Autodesk Inventor part; units mm, degrees
ref_plane "Work Plane1" through (0, 0, 5) normal (0, 0, 1) x (1, 0, 0)
ref_plane "YZ Plane" through (0, 0, 0) normal (1, 0, 0) x (0, 1, 0)
ref_plane "XZ Plane" through (0, 0, 0) normal (0, 1, 0) x (-1, 0, 0)
sketch "Sketch1" plane through (0, 0, 0) normal (0, 0, 1) x (1, 0, 0)
  line L0 (14.6962, 12.74) -> (14.6962, 0) construction
  line L1 (10.61, 12.2) -> (1.53, 12.2)
  arc A0 (1.53, 12.2) -> (0, 10.67) centre (1.53, 10.67) ccw
  line L2 (0, 10.67) -> (0, 1.53)
  arc A1 (0, 1.53) -> (1.53, 0) centre (1.53, 1.53) ccw
  line L3 (1.53, 0) -> (10.61, 0)
  arc A2 (10.61, 0) -> (12.14, 1.53) centre (10.61, 1.53) ccw
  arc A3 (12.14, 10.67) -> (10.61, 12.2) centre (10.61, 10.67) ccw
  line L4 (12.14, 10.67) -> (12.14, 1.53)
  point P0 (0, 0)
  point P1 (0, 0)
  dimension "d10" = 12.74
ref_plane "Work Plane1" through (0, 0, 5) normal (0, 0, 1) x (1, 0, 0)
sketch "Sketch2" plane through (0, 0, 5) normal (0, 0, 1) x (1, 0, 0)
  line L0 (10.88, 12.74) -> (1.8, 12.74)
  line L1 (10.88, 12.74) -> (1.8, 12.74)
  arc A0 (1.8, 12.74) -> (0, 10.94) centre (1.8, 10.94) ccw
  line L2 (0, 10.94) -> (0, 1.8)
  arc A1 (0, 1.8) -> (1.8, 0) centre (1.8, 1.8) ccw
  line L3 (1.8, 0) -> (10.88, 0)
  arc A2 (10.88, 0) -> (12.68, 1.8) centre (10.88, 1.8) ccw
  line L4 (12.68, 1.8) -> (12.68, 10.94)
  arc A3 (12.68, 10.94) -> (10.88, 12.74) centre (10.88, 10.94) ccw
  circle A4 centre (6.34, 6.37) radius 2.8
  line L5 (5.665, 8.395) -> (7.015, 8.395)
  line L6 (7.015, 4.345) -> (5.665, 4.345)
  line L7 (5.665, 4.345) -> (7.015, 8.395) construction
  line L8 (5.665, 8.395) -> (7.015, 4.345) construction
  line L9 (8.365, 5.695) -> (8.365, 7.045)
  line L10 (4.315, 7.045) -> (4.315, 5.695)
  line L11 (4.315, 5.695) -> (8.365, 7.045) construction
  line L12 (8.365, 5.695) -> (4.315, 7.045) construction
  line L13 (4.315, 5.695) -> (5.665, 5.695)
  line L14 (7.015, 5.695) -> (8.365, 5.695)
  line L15 (5.665, 4.345) -> (5.665, 5.695)
  line L16 (5.665, 7.045) -> (5.665, 8.395)
  line L17 (8.365, 7.045) -> (7.015, 7.045)
  line L18 (5.665, 7.045) -> (4.315, 7.045)
  line L19 (7.015, 8.395) -> (7.015, 7.045)
  line L20 (7.015, 5.695) -> (7.015, 4.345)
  point P0 (0, 0)
  dimension "d12" = 5
  dimension "d3" = 5.6
  dimension "d4" = 4.05
  dimension "d5" = 1.35
  dimension "d6" = 4.05
  dimension "d7" = 1.35
extrude "Extrusion3" add sketch "Sketch1" along normal blind 5
sketch "Sketch3" plane through (0, 0, 5) normal (0, 0, 1) x (1, 0, 0)
  line L0 (10.61, 12.47) -> (1.53, 12.47)
  line L1 (10.61, 12.47) -> (1.53, 12.47)
  arc A0 (1.53, 12.47) -> (-0.27, 10.67) centre (1.53, 10.67) ccw
  line L2 (-0.27, 10.67) -> (-0.27, 1.53)
  arc A1 (-0.27, 1.53) -> (1.53, -0.27) centre (1.53, 1.53) ccw
  line L3 (1.53, -0.27) -> (10.61, -0.27)
  arc A2 (10.61, -0.27) -> (12.41, 1.53) centre (10.61, 1.53) ccw
  line L4 (12.41, 1.53) -> (12.41, 10.67)
  arc A3 (12.41, 10.67) -> (10.61, 12.47) centre (10.61, 10.67) ccw
  circle A4 centre (6.07, 6.1) radius 2.8
  line L5 (5.395, 8.125) -> (6.745, 8.125)
  line L6 (6.745, 4.075) -> (5.395, 4.075)
  line L7 (5.395, 4.075) -> (6.745, 8.125) construction
  line L8 (5.395, 8.125) -> (6.745, 4.075) construction
  line L9 (8.095, 5.425) -> (8.095, 6.775)
  line L10 (4.045, 6.775) -> (4.045, 5.425)
  line L11 (4.045, 5.425) -> (8.095, 6.775) construction
  line L12 (8.095, 5.425) -> (4.045, 6.775) construction
  line L13 (4.045, 5.425) -> (5.395, 5.425)
  line L14 (6.745, 5.425) -> (8.095, 5.425)
  line L15 (5.395, 4.075) -> (5.395, 5.425)
  line L16 (5.395, 6.775) -> (5.395, 8.125)
  line L17 (8.095, 6.775) -> (6.745, 6.775)
  line L18 (5.395, 6.775) -> (4.045, 6.775)
  line L19 (6.745, 8.125) -> (6.745, 6.775)
  line L20 (6.745, 5.425) -> (6.745, 4.075)
  line L21 (10.61, 12.2) -> (1.53, 12.2)
  line L22 (0, 10.67) -> (0, 1.53)
  point P0 (0, 0)
  point P1 (-0.27, -0.27)
  point P2 (6.07, 12.2)
  point P3 (0, 6.1)
  point P4 (6.07, 6.1)
  dimension "d14" = 5.6
  dimension "d15" = 4.05
  dimension "d16" = 1.35
  dimension "d17" = 4.05
  dimension "d18" = 1.35
extrude "Extrusion4" add sketch "Sketch3" along normal blind 4.8 contours A4
sketch "Sketch4" plane through (0, 0, 0) normal (0, 0, -1) x (-1, 0, 0)
  line L0 (-13.9436, 0) -> (-13.9436, 2.266)
  line L1 (-15.5559, 0) -> (-15.5559, 6.84)
  line L2 (-1.53, 0) -> (-10.61, 0)
  line L3 (-11.3457, 9.9988) -> (-0.7943, 9.9988) construction
  line L4 (-0.7943, 9.9988) -> (-0.7943, 6.84) construction
  line L5 (-0.7943, 6.84) -> (-11.3457, 6.84) construction
  line L6 (-11.3457, 6.84) -> (-11.3457, 9.9988) construction
  line L7 (-7.4059, 5.3234) -> (-4.7341, 5.3234) construction
  line L8 (-4.7341, 5.3234) -> (-4.7341, 2.266) construction
  line L9 (-4.7341, 2.266) -> (-7.4059, 2.266) construction
  line L10 (-7.4059, 2.266) -> (-7.4059, 5.3234) construction
  spline S0 degree 2 poles (-10.0876, 6.84) (-10.4386, 6.84) (-10.9675, 6.9759) (-11.1949, 7.0748) knots 0 0 0 1 2 2 2
  line L11 (-11.1949, 7.0748) -> (-11.1949, 7.8015)
  line L12 (-11.1949, 7.8015) -> (-11.1257, 7.8015)
  spline S1 degree 2 poles (-11.1257, 7.8015) (-10.8959, 7.6062) (-10.3447, 7.3961) (-10.0852, 7.3961) knots 0 0 0 1 2 2 2
  spline S2 degree 2 poles (-10.0852, 7.3961) (-10.0184, 7.3961) (-9.8034, 7.4258) (-9.7391, 7.4554) knots 0 0 0 1 2 2 2
  spline S3 degree 2 poles (-9.7391, 7.4554) (-9.6601, 7.49) (-9.5488, 7.6161) (-9.5488, 7.7174) knots 0 0 0 1 2 2 2
  spline S4 degree 2 poles (-9.5488, 7.7174) (-9.5488, 7.8336) (-9.7293, 7.977) (-9.8528, 8.0091) knots 0 0 0 1 2 2 2
  spline S5 degree 2 poles (-9.8528, 8.0091) (-10.0086, 8.0511) (-10.362, 8.1228) (-10.5177, 8.1772) knots 0 0 0 1 2 2 2
  spline S6 degree 2 poles (-10.5177, 8.1772) (-10.8712, 8.3007) (-11.1776, 8.7234) (-11.1776, 9.0398) knots 0 0 0 1 2 2 2
  spline S7 degree 2 poles (-11.1776, 9.0398) (-11.1776, 9.4674) (-10.4534, 9.9988) (-9.9097, 9.9988) knots 0 0 0 1 2 2 2
  spline S8 degree 2 poles (-9.9097, 9.9988) (-9.6378, 9.9988) (-9.099, 9.8875) (-8.8864, 9.7936) knots 0 0 0 1 2 2 2
  line L13 (-8.8864, 9.7936) -> (-8.8864, 9.0966)
  line L14 (-8.8864, 9.0966) -> (-8.9532, 9.0966)
  spline S9 degree 2 poles (-8.9532, 9.0966) (-9.1237, 9.2424) (-9.6131, 9.4426) (-9.8701, 9.4426) knots 0 0 0 1 2 2 2
  spline S10 degree 2 poles (-9.8701, 9.4426) (-9.9715, 9.4426) (-10.1297, 9.413) (-10.2186, 9.3734) knots 0 0 0 1 2 2 2
  spline S11 degree 2 poles (-10.2186, 9.3734) (-10.2903, 9.3413) (-10.3941, 9.2128) (-10.3941, 9.1337) knots 0 0 0 1 2 2 2
  spline S12 degree 2 poles (-10.3941, 9.1337) (-10.3941, 9.015) (-10.2285, 8.8791) (-9.9913, 8.8247) knots 0 0 0 1 2 2 2
  spline S13 degree 2 poles (-9.9913, 8.8247) (-9.838, 8.7901) (-9.5538, 8.7234) (-9.3906, 8.6665) knots 0 0 0 1 2 2 2
  spline S14 degree 2 poles (-9.3906, 8.6665) (-9.0743, 8.5504) (-8.7653, 8.1648) (-8.7653, 7.8484) knots 0 0 0 1 2 2 2
  spline S15 degree 2 poles (-8.7653, 7.8484) (-8.7653, 7.3936) (-9.4796, 6.84) (-10.0876, 6.84) knots 0 0 0 1 2 2 2
  line L15 (-7.7866, 6.8944) -> (-7.7866, 9.3635)
  line L16 (-7.7866, 9.3635) -> (-8.6887, 9.3635)
  line L17 (-8.6887, 9.3635) -> (-8.6887, 9.9444)
  line L18 (-8.6887, 9.9444) -> (-6.1182, 9.9444)
  line L19 (-6.1182, 9.9444) -> (-6.1182, 9.3635)
  line L20 (-6.1182, 9.3635) -> (-7.0203, 9.3635)
  line L21 (-7.0203, 9.3635) -> (-7.0203, 6.8944)
  line L22 (-7.0203, 6.8944) -> (-7.7866, 6.8944)
  spline S16 degree 2 poles (-3.4587, 8.9829) (-3.4587, 8.7703) (-3.5947, 8.3848) (-3.7207, 8.2562) knots 0 0 0 1 2 2 2
  spline S17 degree 2 poles (-3.7207, 8.2562) (-3.7973, 8.1747) (-3.9852, 8.0412) (-4.0964, 7.9943) knots 0 0 0 1 2 2 2
  spline S18 degree 2 poles (-4.0964, 7.9943) (-4.2101, 7.9473) (-4.4746, 7.8929) (-4.6377, 7.8929) knots 0 0 0 1 2 2 2
  line L23 (-4.6377, 7.8929) -> (-5.0381, 7.8929)
  line L24 (-5.0381, 7.8929) -> (-5.0381, 6.8944)
  line L25 (-5.0381, 6.8944) -> (-5.8043, 6.8944)
  line L26 (-5.8043, 6.8944) -> (-5.8043, 9.9444)
  line L27 (-5.8043, 9.9444) -> (-4.6204, 9.9444)
  spline S19 degree 2 poles (-4.6204, 9.9444) (-4.3584, 9.9444) (-3.9753, 9.848) (-3.8196, 9.7442) knots 0 0 0 1 2 2 2
  spline S20 degree 2 poles (-3.8196, 9.7442) (-3.6466, 9.628) (-3.4587, 9.2474) (-3.4587, 8.9829) knots 0 0 0 1 2 2 2
  spline S21 degree 2 poles (-4.2447, 8.9631) (-4.2447, 9.0941) (-4.3683, 9.2795) (-4.4523, 9.3141) knots 0 0 0 1 2 2 2
  spline S22 degree 2 poles (-4.4523, 9.3141) (-4.5611, 9.3611) (-4.7588, 9.3759) (-4.9293, 9.3759) knots 0 0 0 1 2 2 2
  line L28 (-4.9293, 9.3759) -> (-5.0381, 9.3759)
  line L29 (-5.0381, 9.3759) -> (-5.0381, 8.4614)
  line L30 (-5.0381, 8.4614) -> (-4.9837, 8.4614)
  spline S23 degree 2 poles (-4.9837, 8.4614) (-4.8774, 8.4614) (-4.6846, 8.4663) (-4.613, 8.4787) knots 0 0 0 1 2 2 2
  spline S24 degree 2 poles (-4.613, 8.4787) (-4.5512, 8.4886) (-4.4152, 8.5479) (-4.3782, 8.585) knots 0 0 0 1 2 2 2
  spline S25 degree 2 poles (-4.3782, 8.585) (-4.2991, 8.6591) (-4.2447, 8.8247) (-4.2447, 8.9631) knots 0 0 0 1 2 2 2
  line L31 (-2.4626, 6.8944) -> (-2.4626, 9.3635)
  line L32 (-2.4626, 9.3635) -> (-3.3648, 9.3635)
  line L33 (-3.3648, 9.3635) -> (-3.3648, 9.9444)
  line L34 (-3.3648, 9.9444) -> (-0.7943, 9.9444)
  line L35 (-0.7943, 9.9444) -> (-0.7943, 9.3635)
  line L36 (-0.7943, 9.3635) -> (-1.6964, 9.3635)
  line L37 (-1.6964, 9.3635) -> (-1.6964, 6.8944)
  line L38 (-1.6964, 6.8944) -> (-2.4626, 6.8944)
  line L39 (-4.8181, 2.9852) -> (-5.2309, 2.9852)
  line L40 (-5.2309, 2.9852) -> (-5.2309, 2.266)
  line L41 (-5.2309, 2.266) -> (-5.9699, 2.266)
  line L42 (-5.9699, 2.266) -> (-5.9699, 2.9852)
  line L43 (-5.9699, 2.9852) -> (-7.3145, 2.9852)
  line L44 (-7.3145, 2.9852) -> (-7.3145, 3.5537)
  line L45 (-7.3145, 3.5537) -> (-5.9946, 5.3234)
  line L46 (-5.9946, 5.3234) -> (-5.2309, 5.3234)
  line L47 (-5.2309, 5.3234) -> (-5.2309, 3.5339)
  line L48 (-5.2309, 3.5339) -> (-4.8181, 3.5339)
  line L49 (-4.8181, 3.5339) -> (-4.8181, 2.9852)
  line L50 (-5.9699, 3.5339) -> (-5.9699, 4.572)
  line L51 (-5.9699, 4.572) -> (-6.7435, 3.5339)
  line L52 (-6.7435, 3.5339) -> (-5.9699, 3.5339)
  point P0 (0, 0)
  point P1 (-6.07, 0)
  point P2 (-6.07, 2.266)
  point P3 (-6.07, 6.84)
  point P4 (-6.07, 6.84)
  point P5 (-6.07, 2.266)
  dimension "d21" = 2.266
  dimension "d22" = 6.84
sketch "Sketch5" plane through (0, 0, 0) normal (0, 0, -1) x (-1, 0, 0)
  point P0 (0, 0)
extrude "Extrusion5" add sketch "Sketch4" along normal blind 0.9
properties part number "IPC STPT 4 key"
Can you work these out from the model? Positions are in its coordinate system, mm. A direction names the side the tool comes from. Give positions to 0.01 mm unless a question says otherwise; leave off trailing zeros. Order: outer loops, then holes, each group sorted by start corner. A loop starts at its lowest first (then second) coordinate and runs counter-clockwise, first axis right, second up. Notation, with made-up numbers: (46, 60.25) - (83, 60.25) arc R36 cw to (83, 99.25) - close; hole circle Ø2 at (85.5, 37). An arc over 180 degrees is marked (long way). Use a Markdown table: item, result. Add a question column.
Q1. If we mould it in two halves opening along Y, with no side actions, what happens to faces 6 (the flat face through (1.696, 8.1, -0.4)), 7 (the flat face through (5.038, 8.9, -0.4)), 8 (the cylindrical face through (11.704, 0.46, 2.465)), 9 (the cylindrical face through (5.463, 8.833, 7.366))? For each: released by +Y, released by -Y, zero draft, split by the parting line, or undercut.
Q2. If we section it at D-D on y = 6.1: Write out the boundary of the cut face in (x, z) (3 decimals).
Q3. If we section it at B-B on y = 2.5: Write out the boundary of the cut face in (x, z), plus the area to 3 significant figures.
Q4. On a 3-axis mill with a long thin cutter (end or side, diameter ignored), from which of +Z, -Z, +X, -X, +Y, -Y can I reach the whole of each face in a straight line? I mean faces 1 (the flat face through (6, 0, 2)), 2 (the flat face through (8.095, 6, 7)), 3 (the flat face through (5.2, 9.944, -0.4)), 4 (the flat face through (5.231, 4.4, -0.4)), 5 (the flat face through (2.463, 8.1, -0.4)). Say none if no direction works.
Q5. I'm going to push flat-ended pins straight in: pin 1 (2 mm diameter, centred on x = 7, z = 8, fed in from +Y); pin 2 (1 mm diameter, centred on x = 2.5, y = 9.5, fed in from +Z); pin 3 (0.6 mm diameter, centred on y = 7.5, z = -0.5, fed in from +X). Where does each tip first touch, or does it pass through?
Q6. If we section it at A-A on z = 5.25: Write out the boundary of the cut face in (x, y) (3 decimals), plus the area to 3 significant figures.
Q7. Please list where these lines run through material, in increasing order: line 1 along Z through (x, y) = (4.75, 2); line 2 along Z through (x, y) = (2.5, 9.75); line 3 along X through (y, z) = (10.75, 0.25).
Answers follow:
| question | item | result |
|---|---|---|
| 1 | face 6 | zero draft |
| 1 | face 7 | undercut |
| 1 | face 8 | released by -Y |
| 1 | face 9 | split by the parting line |
| 2 | outline | (0, 0) - (12.14, 0) - (12.14, 5) - (8.87, 5) - (8.87, 9.8) - (8.095, 9.8) - (8.095, 5) - (4.045, 5) - (4.045, 9.8) - (3.27, 9.8) - (3.27, 5) - (0, 5) - close |
| 3 | outline | (0, 0) - (5.23, 0) - (5.23, -0.9) - (5.97, -0.9) - (5.97, 0) - (12.14, 0) - (12.14, 5) - (0, 5) - close |
| 3 | area | 61.4 mm^2 |
| 4 | face 1 | +Z, -Z, +X, -X, -Y |
| 4 | face 2 | +Z |
| 4 | face 3 | -Z, -X, +Y |
| 4 | face 4 | -Z, -X |
| 4 | face 5 | -Z, -Y |
| 5 | pin 1 | stops at y = 8.9 |
| 5 | pin 2 | stops at z = 5 |
| 5 | pin 3 | stops at x = 11.19 |
| 6 | outline | circle Ø5.6 at (6.07, 6.1); hole (4.045, 5.425) - (5.395, 5.425) - (5.395, 4.075) - (6.745, 4.075) - (6.745, 5.425) - (8.095, 5.425) - (8.095, 6.775) - (6.745, 6.775) - (6.745, 8.125) - (5.395, 8.125) - (5.395, 6.775) - (4.045, 6.775) - close |
| 6 | area | 15.5 mm^2 |
| 7 | line 1 | z = 0 to 5 |
| 7 | line 2 | z = -0.9 to 5 |
| 7 | line 3 | x = 0 to 12.14 |
